from build123d import *

# Parameters (mm, degrees)
SKETCH2_W           = 25.4
SKETCH2_H           = 25.4
SKETCH2_W_2         = 22.86
SKETCH2_H_2         = 22.86
BOSS_EXTRUDE1_DEPTH = 63.5
SKETCH3_R           = 2.413
CUT_EXTRUDE1_DEPTH  = 70.560764803
SKETCH4_R           = 2.413
CUT_EXTRUDE2_DEPTH  = 70.560764803


with BuildPart() as part:
    # Sketch2 → Boss-Extrude1 (new body)
    with BuildSketch(Plane(origin=(0, 0, 0), x_dir=(1, 0, 0), z_dir=(0, 1, 0))):
        Rectangle(SKETCH2_W, SKETCH2_H)
        with Locations((0, 0.262548077)):
            Rectangle(SKETCH2_W_2, SKETCH2_H_2, mode=Mode.SUBTRACT)
    extrude(amount=BOSS_EXTRUDE1_DEPTH)

    # Sketch3 → Cut-Extrude1 (cut, through all)
    with BuildSketch(Plane(origin=(0, 0, -12.7), x_dir=(-1, 0, 0), z_dir=(0, 0, -1))):
        with Locations((0, 57.15)):
            Circle(SKETCH3_R)
        with Locations((0, 44.45)):
            Circle(SKETCH3_R)
        with Locations((0, 31.75)):
            Circle(SKETCH3_R)
        with Locations((0, 19.05)):
            Circle(SKETCH3_R)
        with Locations((0, 6.35)):
            Circle(SKETCH3_R)
        with Locations((0, -6.35)):
            Circle(SKETCH3_R)
    extrude(amount=-CUT_EXTRUDE1_DEPTH, mode=Mode.SUBTRACT)

    # Sketch4 → Cut-Extrude2 (cut, through all)
    with BuildSketch(Plane(origin=(12.7, 0, 0), x_dir=(0, 0, -1), z_dir=(1, 0, 0))):
        with Locations((0, 57.15)):
            Circle(SKETCH4_R)
        with Locations((0, 44.45)):
            Circle(SKETCH4_R)
        with Locations((0, 31.75)):
            Circle(SKETCH4_R)
        with Locations((0, 19.05)):
            Circle(SKETCH4_R)
        with Locations((0, 6.35)):
            Circle(SKETCH4_R)
        with Locations((0, -6.35)):
            Circle(SKETCH4_R)
    extrude(amount=-CUT_EXTRUDE2_DEPTH, mode=Mode.SUBTRACT)


solid = part.part
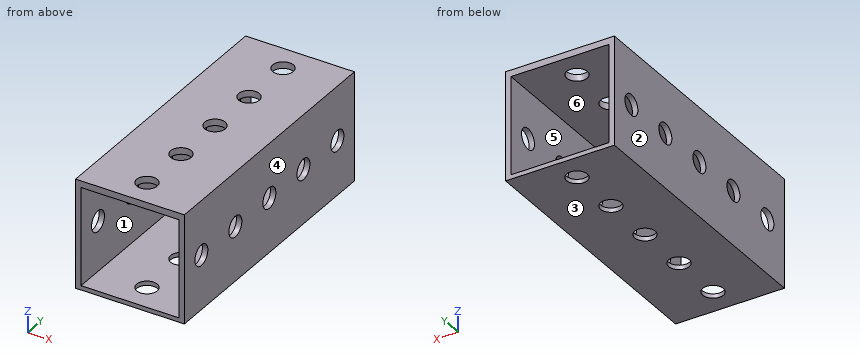
Build history of the part. All positions in model axes, mm. Face numbers are marked on the shaded views. A direction names the side the tool comes from. Round coordinates to 2 decimals unless told otherwise and drop trailing zeros. Write each loop counter-clockwise with the first axis right and the second up, starting at its lowest first coordinate (ties: lowest second). Pieces come first, ordered by that corner, then holes. Notation, with made-up numbers: (-37.5, -32.5) - (0.5, -32.5) arc R18 ccw to (0.5, 2.5) - close; hole circle Ø1 at (85, -33). An arc over 180 degrees is marked (long way). One line per question, with ' | ' between items.
1. Band-saw the part on B-B, the plane x = -5. Write the cut outline in (y, z), and give its area (3 significant figures).
Results are:
outline: (0, -12.7) - (63.5, -12.7) - (63.5, -11.69) - (0, -11.69) - close; (0, 11.17) - (63.5, 11.17) - (63.5, 12.7) - (0, 12.7) - close | area: 161 mm^2
2. Mould opens along Z. For the marked faces 3, 4, 5 and 6 say: released by +Z, released by -Z, zero draft, split by the parting line, or undercut.
Results are:
face 3: released by -Z | face 4: zero draft | face 5: undercut | face 6: undercut
3. Drill centre lines: line 1 along Y through (x, z) = (0, -12.05); line 2 along Z through (x, y) = (-5, 4); line 3 along X through (y, z) = (29, -4.5). Where is each one in solid material? Low to high. Write a range as from..to.
Results are:
line 1: 0..3.94, 8.76..16.64, 21.46..29.34, 34.16..42.04, 46.86..54.74, 59.56..63.5 | line 2: -12.7..-11.69, 11.17..12.7 | line 3: -12.7..-11.43, 11.43..12.7
4. Band-saw the part on C-C, the plane y = 11.5. Write the cut outline in (x, z), and give its area (3 significant figures).
Results are:
outline: (-12.7, -12.7) - (12.7, -12.7) - (12.7, 12.7) - (-12.7, 12.7) - close; hole (-11.43, -11.69) - (11.43, -11.69) - (11.43, 11.17) - (-11.43, 11.17) - close | area: 123 mm^2
5. Band-saw the part on A-A, the plane y = 19.05. Write the cut outline in (x, z), and give its area (3 significant figures).
Results are:
outline: (-12.7, -12.7) - (-2.41, -12.7) - (-2.41, -11.69) - (-11.43, -11.69) - (-11.43, -2.41) - (-12.7, -2.41) - close; (-12.7, 2.41) - (-11.43, 2.41) - (-11.43, 11.17) - (-2.41, 11.17) - (-2.41, 12.7) - (-12.7, 12.7) - close; (2.41, -12.7) - (12.7, -12.7) - (12.7, -2.41) - (11.43, -2.41) - (11.43, -11.69) - (2.41, -11.69) - close; (2.41, 11.17) - (11.43, 11.17) - (11.43, 2.41) - (12.7, 2.41) - (12.7, 12.7) - (2.41, 12.7) - close | area: 98.1 mm^2
6. Drop a flat-ended pin along its axis: pin 1 Ø5.5 at (y, z) = (31.75, 0) entering from -X. Give the stop position or say it passes through.
Results are:
pin 1: x = -12.7
7. Tool access for the marked faces 1 and 2: list every direction of +Z, -Z, +X, -X, +Y, -Y with a clear straight run to the whole face (end or side of a thin tool).
Results are:
face 1: +Y, -Y | face 2: +Z, -Z, -X, +Y, -Y
8. Band-saw the part on D-D, the plane z = 7.75. Write the cut outline in (x, y), and give its area (3 significant figures).
Results are:
outline: (-12.7, 0) - (-11.43, 0) - (-11.43, 63.5) - (-12.7, 63.5) - close; (11.43, 0) - (12.7, 0) - (12.7, 63.5) - (11.43, 63.5) - close | area: 161 mm^2
